Could you check a few things on this drawing? It's one solid part, dimensions in mm from its lowest x, y, z. Round coordinates to 2 decimals unless told otherwise and drop trailing zeros. Loops run counter-clockwise (first coordinate to the right, second up) from the corner with the lowest first, then second, coordinate; pieces in that order, holes last. Notation, with made-up numbers: (-38, -20) -> (15, -20) arc R10 ccw to (15, -15) -> close; hole circle Ø11 at (-40, 67.25). An arc over 180 degrees is marked (long way). Put each result on its own line as item: value. Start each with the question number.
1. Imagine slicing it at A-A, the plane x = 29. Please give me the cut outline in (y, z).
2. I'm going to push flat-ended pins straight in: P1, Ø1.5, axis at x = 57.5, z = 96.5, coming from the +Y side; P2, Ø4, axis at x = 53, z = 65.5, coming from the -Y side; P3, Ø17.5, axis at x = 32, z = 102, coming from the -Y side. Where does each tip first touch, or does it pass through?
3. If we mould it in two halves opening along X, with no side actions, what happens to the marked faces 1 and 2? For each: pulls with the +X half, pulls with the -X half, needs draft (parallel to the pull), parting line crosses it, or undercut.
4. Imagine slicing it at C-C, the plane y = 6.5. Please give me the cut outline in (x, z).
5. Imagine slicing it at D-D, the plane x = 89.5. Please give me the cut outline in (y, z), and give its area (3 significant figures).
6. I need wall thicknesses on line 1 (Y direction, x = 43.5, z = 109); line 2 (Y direction, x = 81, z = 120); line 3 (X direction, y = 10.5, z = 21.5). Which ranges of each line are inside material? Lowest first, please. Write a range as [from, to].
7. Imagine slicing it at B-B, the plane z = 97. Please give me the cut outline in (x, y).
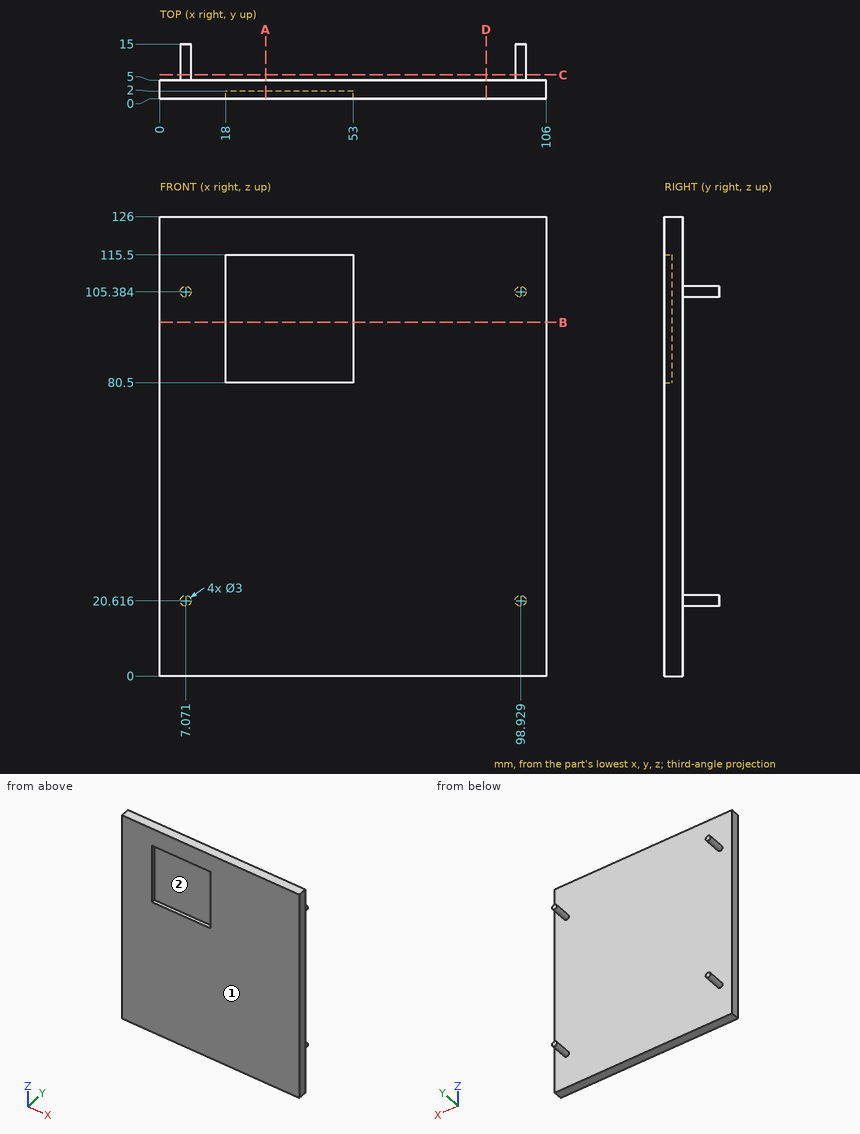
Entries:
1. outline: (0, 0) -> (5, 0) -> (5, 126) -> (0, 126) -> (0, 115.5) -> (2, 115.5) -> (2, 80.5) -> (0, 80.5) -> close
2. P1: y = 5
2. P2: y = 0
2. P3: y = 2
3. face 1: needs draft
3. face 2: undercut
4. outline: circle Ø3 at (7.07, 20.62); circle Ø3 at (7.07, 105.38); circle Ø3 at (98.93, 20.62); circle Ø3 at (98.93, 105.38)
5. outline: (0, 0) -> (5, 0) -> (5, 126) -> (0, 126) -> close
5. area: 630 mm^2
6. line 1: [2, 5]
6. line 2: [0, 5]
6. line 3: [5.86, 8.28], [97.72, 100.14]
7. outline: (0, 0) -> (18, 0) -> (18, 2) -> (53, 2) -> (53, 0) -> (106, 0) -> (106, 5) -> (0, 5) -> close
